Read the model definition and answer for the solid it produces. Units are mm, in the model's axes. A direction names the side the tool comes from. Coordinates: 2 decimals unless noted, no trailing zeros. Write each loop counter-clockwise with the first axis right and the second up, starting at its lowest first coordinate (ties: lowest second). Pieces come first, ordered by that corner, then holes.
from build123d import *

# Parameters (mm, degrees)
SKETCH2_R           = 16.052702668
BOSS_EXTRUDE1_DEPTH = 203
CUT_EXTRUDE1_DEPTH  = 476


with BuildPart() as part:
    # Sketch2 → Boss-Extrude1 (new body)
    with BuildSketch(Plane.XY):
        Circle(SKETCH2_R)
    extrude(amount=-BOSS_EXTRUDE1_DEPTH)

    # Sketch5 → Cut-Extrude1 (cut)
    with BuildSketch(Plane.XY):
        Polygon((6.249490897, -11.192871263), (12.818056304, -0.184217754), (6.568565406, 11.008653509), (-6.249490897, 11.192871263), (-12.818056304, 0.184217754), (-6.568565406, -11.008653509), align=None)
    extrude(amount=-CUT_EXTRUDE1_DEPTH, mode=Mode.SUBTRACT)


solid = part.part
Item 1: Find the intervals of material crossed by probe 1 along X at (y, z) = (-6, -174); probe 2 along Y at (x, z) = (-9, -144); probe 3 along Y at (x, z) = (6, -183), in increasing order.
Item 2: The part is cut by section A-A (z = -39). Give the vertices of the cut face in (x, y), and give its area (3 significant figures).
Item 3: The part is cut by section B-B (x = 9). Give the vertices of the cut face in (y, z).
Item 4: Determine the mould class of faces 3 (the flat face through (9.74, 5.33, -100.08)), 4 (the flat face through (-11, 4, 0)), 5 (the cylindrical face through (-3.48, -15.67, -100.08)) for opening direction X: +X half, -X half, draft (parallel to the pull), parting line (faces both ways), or undercut.
Item 5: For faces 1 (the flat face through (-11, 4, -203)), 2 (the flat face through (-9.488, 5.766, -100.079)), determine the directions among +Z, -Z, +X, -X, +Y, -Y from which every point of the face is accessible in a straight line to the end or side of a thin tool.
Item 6: The part is cut by section C-C (y = -9). Give the vertices of the cut face in (x, z).
Item 7: Given pin 1 (6 mm diameter, centred on y = -5, z = -83, fed in from +X); pin 2 (5 mm diameter, centred on y = 3.5, z = -39.5, fed in from +X); pin 3 (10 mm diameter, centred on x = -11.5, z = -46, fed in from +Y), each flat-ended and moving along its own axis, determine where each tip first touches the part or whether it passes through.
Item 8: The part is cut by section D-D (y = 14). Give the vertices of the cut face in (x, z).
Answer:
1. probe 1: x = -14.89 to -9.37, 9.35 to 14.89
1. probe 2: y = -13.29 to -6.65, 6.58 to 13.29
1. probe 3: y = -14.89 to -11.19, 11.02 to 14.89
2. outline: circle Ø32.11 at (0, 0); hole (-12.82, 0.18) - (-6.57, -11.01) - (6.25, -11.19) - (12.82, -0.18) - (6.57, 11.01) - (-6.25, 11.19) - close
2. area: 383 mm2
3. outline: (-13.29, -203) - (-6.58, -203) - (-6.58, 0) - (-13.29, 0) - close; (6.65, -203) - (13.29, -203) - (13.29, 0) - (6.65, 0) - close
4. face 3: undercut
4. face 4: draft
4. face 5: parting line
5. face 1: -Z, +X, -X, +Y, -Y
5. face 2: +Z, -Z
6. outline: (-13.29, -203) - (-7.69, -203) - (-7.69, 0) - (-13.29, 0) - close; (7.56, -203) - (13.29, -203) - (13.29, 0) - (7.56, 0) - close
7. pin 1: stops at x = 15.93
7. pin 2: stops at x = 16.02
7. pin 3: stops at y = 14.68
8. outline: (-7.85, -203) - (7.85, -203) - (7.85, 0) - (-7.85, 0) - close
